```python
from build123d import *

# Parameters (mm, degrees)
SKETCH2_W           = 65
SKETCH2_H           = 10
BOSS_EXTRUDE1_DEPTH = 5
FILLET1_R           = 2
FILLET2_R           = 2
SKETCH3_R           = 2
CUT_EXTRUDE1_DEPTH  = 15
LPATTERN1_COUNT     = 5
LPATTERN1_PITCH     = 12
SKETCH4_W           = 7.213630723
SKETCH4_H           = 10
BOSS_EXTRUDE2_DEPTH = 60
SKETCH5_R           = 2
CUT_EXTRUDE2_DEPTH  = 60
LPATTERN2_COUNT     = 3
LPATTERN2_PITCH     = 12
LPATTERN2_COL_COUNT = 2
LPATTERN2_COL_PITCH = 12
FILLET3_R           = 2


with BuildPart() as part:
    # Sketch2 → Boss-Extrude1 (new body)
    with BuildSketch(Plane(origin=(0, 0, 0), x_dir=(1, 0, 0), z_dir=(0, 1, 0))):
        with Locations((-5.357142857, 0.803571429)):
            Rectangle(SKETCH2_W, SKETCH2_H)
    extrude(amount=BOSS_EXTRUDE1_DEPTH)

    # Fillet1
    fillet1_edges = [part.edges().sort_by_distance(p)[0] for p in [
        (-37.857142857, 2.5, 4.196428571),
    ]]
    fillet(fillet1_edges, radius=FILLET1_R)

    # Fillet2
    fillet2_edges = [part.edges().sort_by_distance(p)[0] for p in [
        (-37.857142857, 2.5, -5.803571429),
    ]]
    fillet(fillet2_edges, radius=FILLET2_R)

    # Sketch3 → Cut-Extrude1 (cut)
    with BuildSketch(Plane(origin=(0, 5, 0), x_dir=(1, 0, 0), z_dir=(0, 1, 0))):
        with Locations(Location((13.625145437, 0.803571429, 0), (0, 0, 270))):
            Circle(SKETCH3_R)
    cut_extrude1 = extrude(amount=-CUT_EXTRUDE1_DEPTH, mode=Mode.SUBTRACT)

    # LPattern1: Cut-Extrude1 ×5
    with Locations(*[(-i * LPATTERN1_PITCH, 0, 0) for i in range(1, LPATTERN1_COUNT)]):
        add(cut_extrude1, mode=Mode.SUBTRACT)

    # Sketch4 → Boss-Extrude2 (add)
    with BuildSketch(Plane(origin=(0, 5, 0), x_dir=(1, 0, 0), z_dir=(0, 1, 0))):
        with Locations((23.536041782, 0.803571429)):
            Rectangle(SKETCH4_W, SKETCH4_H)
    extrude(amount=BOSS_EXTRUDE2_DEPTH)

    # Sketch5 → Cut-Extrude2 (cut)
    with BuildSketch(Plane.ZY.offset(-19.92922642)):
        with Locations((-0.803571429, 28.14)):
            Circle(SKETCH5_R)
    cut_extrude2 = extrude(amount=-CUT_EXTRUDE2_DEPTH, mode=Mode.SUBTRACT)

    # LPattern2: Cut-Extrude2 ×3
    with Locations(*[(0, i * LPATTERN2_PITCH, 0) for i in range(1, LPATTERN2_COUNT)]):
        add(cut_extrude2, mode=Mode.SUBTRACT)

    # LPattern2 col: Cut-Extrude2 ×2
    with Locations(*[(0, -i * LPATTERN2_COL_PITCH, 0) for i in range(1, LPATTERN2_COL_COUNT)]):
        add(cut_extrude2, mode=Mode.SUBTRACT)

    # Fillet3
    fillet3_edges = [part.edges().sort_by_distance(p)[0] for p in [
        (27.142857143, 65, -0.803571429),
        (23.536041781, 65, -5.803571429),
        (19.92922642, 65, -0.803571429),
        (23.536041781, 65, 4.196428571),
    ]]
    fillet(fillet3_edges, radius=FILLET3_R)


solid = part.part
```
Design review of the part built by this model. Coordinates are the model's own, in mm. A direction names the side the tool comes from. Coordinates: 2 decimals unless noted, no trailing zeros. Order: outer loops, then holes, each group sorted by start corner. A loop starts at its lowest first (then second) coordinate and runs counter-clockwise, first axis right, second up. Notation, with made-up numbers: (67, -39.5) -> (91, -39.5) arc R22 ccw to (91, -28.5) -> close; hole circle Ø6 at (27, 13.5). An arc over 180 degrees is marked (long way). One line per item, written item: value. Start each with the question number.
Q1. For probe 1 along Y at (x, z) = (24.5, 0.5); probe 2 along Y at (x, z) = (7.5, 2); probe 3 along X at (y, z) = (20, 3.25), list the stretches that pass through material, from the lowest coordinate up.
Q2. Tool access review of faces 4 (the cylindrical face through (-37.29, 2.54, -5.2)), 5 (the flat face through (-9, 5, -3)): name each direction out of +Z, -Z, +X, -X, +Y, -Y from which nothing blocks a thin tool from reaching the whole face with its end or side.
Q3. Take a section at B-B, the plane x = 14.5. State the section outline as (y, z) points, then the cut area to 3 significant figures.
Q4. Take a section at A-A, the plane y = 52.14. State the section outline as (x, z) points, then the cut area to 3 significant figures.
Q5. Insertion check: pin 1 Ø3 at (y, z) = (36, 1) entering from -X; pin 2 Ø3 at (x, z) = (3.5, 1.5) entering from +Y. Each pin has a flat end and moves straight along its axis. Give the tip position at first contact, or say it passes through.
Q6. Mouldability with a two-part tool opening along Y and no side actions: class faces 1 (the cylindrical face through (20.5, 64.4, -0.9)), 2 (the cylindrical face through (23.49, 14.19, -1.24)), 3 (the cylindrical face through (11.673, 2.535, -1.237)) as pulls with the +Y half, pulls with the -Y half, needs draft (parallel to the pull), parting line crosses it, or undercut.
Values follow:
1. probe 1: y = 0 to 14.62, 17.66 to 26.62, 29.66 to 38.62, 41.66 to 50.62, 53.66 to 65
1. probe 2: y = 0 to 5
1. probe 3: x = 19.93 to 27.14
2. face 4: -Z, -X, +Y, -Y
2. face 5: +Z, -Z, -X, +Y
3. outline: (0, -5.8) -> (5, -5.8) -> (5, -2.6) -> (0, -2.6) -> close; (0, 0.99) -> (5, 0.99) -> (5, 4.2) -> (0, 4.2) -> close
3. area: 32.0 mm2
4. outline: (19.93, -5.8) -> (27.14, -5.8) -> (27.14, -2.8) -> (19.93, -2.8) -> close; (19.93, 1.2) -> (27.14, 1.2) -> (27.14, 4.2) -> (19.93, 4.2) -> close
4. area: 43.3 mm2
5. pin 1: stops at x = 19.93
5. pin 2: stops at y = 5
6. face 1: pulls with the +Y half
6. face 2: undercut
6. face 3: needs draft
